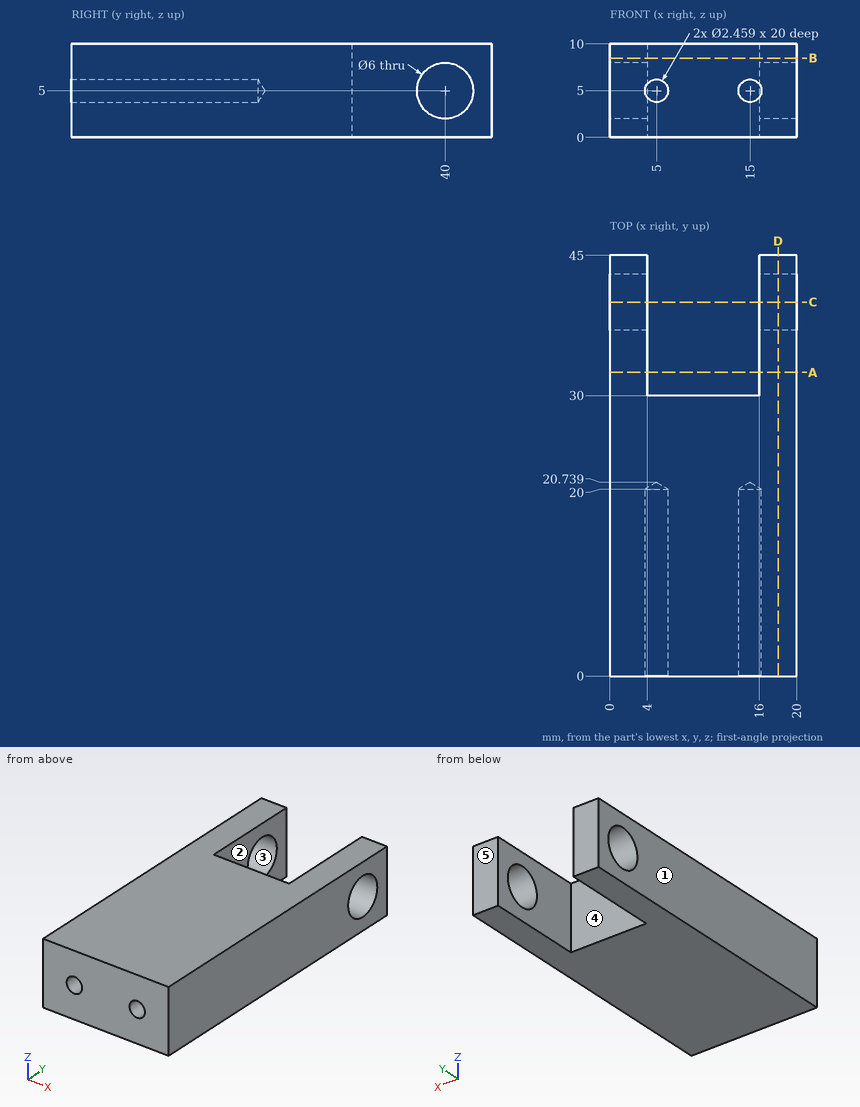
For this review, use the dimensioned drawing (mm, ordinates from the lowest corner) and the shaded views. A direction names the side the tool comes from. Give positions to 0.01 mm unless a question says otherwise; leave off trailing zeros. Write each loop counter-clockwise with the first axis right and the second up, starting at its lowest first coordinate (ties: lowest second). Pieces come first, ordered by that corner, then holes. Notation, with made-up numbers: M 52,-18.75 L 100,-18.75 A34 ccw 100,15.25 Z; hole C -33,12 d6. An arc over 180 degrees is marked long. Answer as a JSON object with one key per item and string values. Group by question number.
Item 1: Tool access review of the marked faces 4 and 5: name each direction out of +Z, -Z, +X, -X, +Y, -Y from which nothing blocks a thin tool from reaching the whole face with its end or side.
Item 2: Consider section A-A on y = 32.5. Write out the cut boundary in (x, z).
Item 3: For pin 1 Ø5 at (x, z) = (10, 4) entering from +Y, flat-tipped, find the tip position at first contact; note if it passes through.
Item 4: For probe 1 along X at (y, z) = (4, 5); probe 2 along Z at (x, y) = (5, 7.5); probe 3 along Z at (x, y) = (1.85, 40), list the stretches that pass through material, from the lowest coordinate up. Write a range as [from, to].
Item 5: Consider section C-C on y = 40. Write out the cut boundary in (x, z), plus the area to 3 significant figures.
Item 6: Draft analysis for pull direction X (two halves, no side actions). For the marked faces 1, 2 and 3, state which applies: +X half, -X half, draft (parallel to the pull), parting line (faces both ways), or undercut.
Item 7: Consider section B-B on z = 8.5. Write out the cut boundary in (x, y), plus the area to 3 significant figures.
Item 8: Consider section D-D on x = 18. Write out the cut boundary in (y, z), plus the area to 3 significant figures.
Check result:
{
 "1": {"face 4": "+Z, -Z, +Y", "face 5": "+Z, -Z, +X, -X, +Y"},
 "2": {"outline": "M 0,0 L 4,0 L 4,10 L 0,10 Z; M 16,0 L 20,0 L 20,10 L 16,10 Z"},
 "3": {"pin 1": "stops at y = 30"},
 "4": {"probe 1": "x = [0, 3.77], [6.23, 13.77], [16.23, 20]", "probe 2": "z = [0, 3.77], [6.23, 10]", "probe 3": "z = [0, 2], [8, 10]"},
 "5": {"outline": "M 0,0 L 4,0 L 4,2 L 0,2 Z; M 0,8 L 4,8 L 4,10 L 0,10 Z; M 16,0 L 20,0 L 20,2 L 16,2 Z; M 16,8 L 20,8 L 20,10 L 16,10 Z", "area": "32.0 mm^2"},
 "6": {"face 1": "-X half", "face 2": "undercut", "face 3": "draft"},
 "7": {"outline": "M 0,0 L 20,0 L 20,45 L 16,45 L 16,30 L 4,30 L 4,45 L 0,45 Z", "area": "720 mm^2"},
 "8": {"outline": "M 0,0 L 45,0 L 45,10 L 0,10 Z; hole C 40,5 d6", "area": "422 mm^2"}
}
